Check sheet for the modelled part. Datum: model origin and axes. Units: mm. A direction names the side the tool comes from. Coordinates: 2 decimals unless noted, no trailing zeros. Loops run counter-clockwise (first coordinate to the right, second up) from the corner with the lowest first, then second, coordinate; pieces in that order, holes last. Notation, with made-up numbers: M 44,20 L 56,20 A23 ccw 56,36 Z; hole C 79.5,47 d7. An arc over 180 degrees is marked long. Use CSV: the item, a comma, the result in double quotes. Start each with the question number.
(1) Go/stop test with flat-tipped pins: pin 1 Ø1.6 at (y, z) = (-1, -3.5) entering from +X; pin 2 Ø5 at (x, z) = (12, 5) entering from -Y; pin 3 Ø0.7 at (x, y) = (49, -1) entering from +Z. Record where each tip stops, or that it passes through.
(2) Section check B-B on z = -1. Record the cut outline in (x, y) (3 decimals), and give its area (3 significant figures).
(3) Draft check along Z on faces 4 (the flat face through (62.8, -0.6, -4.3)), 5 (the flat face through (34, -6, -7)), 6 (the cylindrical face through (1.797, -12.913, -6.63)). Enter one of: pulls with the +Z half, pulls with the -Z half, needs draft (parallel to the pull), parting line crosses it, or undercut.
(4) Scan lines: line 1 (Z direction, x = 55.5, y = -2.5); line 2 (Y direction, x = 30, z = 3). Record each from-to range of solid material in increasing order.
(5) Section check C-C on x = 3.95. Give the number of separate pieces and of enclosed holes in the cut face, and give its area (3 significant figures).
(6) Section check A-A on y = -4.3. Record the cut outline in (x, z), and give its area (3 significant figures).
(7) Set-up check for faces 1 (the flat face through (18.986, -11.146, 6.63)), 2 (the flat face through (53, -1, 2.5)), 3 (the flat face through (51.823, -10.222, -6.62)): record each of +Z, -Z, +X, -X, +Y, -Y from which the full face is reachable in a straight line by a thin tool's end or side.
from build123d import *

# Parameters (mm, degrees)
BOSS_EXTRUDE1_DEPTH = 7
FILLET1_R           = 2
FILLET2_R           = 4
SHELL1_T            = -0.75
SKETCH4_R           = 1.5
CUT_EXTRUDE1_DEPTH  = 71.716642035
CUT_EXTRUDE2_DEPTH  = 14
CUT_EXTRUDE3_DEPTH  = 71.716642035


with BuildPart() as part:
    # Sketch3 → Boss-Extrude1 (new, symmetric)
    with BuildSketch(Plane.XY):
        with BuildLine():
            Line((67, 0), (68.2, -9))
            Line((68.2, -9), (1.2, -14))
            Line((1.2, -14), (0, 0))
            ThreePointArc((0, 0), (33.5, -1), (67, 0))
        make_face()
        with BuildLine():
            ThreePointArc((1.2, -14), (-0.147259987, -7.064050856), (0, 0))
            Line((0, 0), (1.2, -14))
        make_face()
    extrude(amount=BOSS_EXTRUDE1_DEPTH, both=True)

    # Fillet1
    fillet1_edges = [part.edges().sort_by_distance(p)[0] for p in [
        (33.5, -1, 7),
        (33.5, -1, -7),
        (68.2, -9, 0),
    ]]
    fillet(fillet1_edges, radius=FILLET1_R)

    # Fillet2
    fillet2_edges = [part.edges().sort_by_distance(p)[0] for p in [
        (1.2, -14, 0),
    ]]
    fillet(fillet2_edges, radius=FILLET2_R)

    # Shell1
    shell1_openings = [part.faces().sort_by_distance(p)[0] for p in [
        (67.467137389, -3.503530417, 0),
        (67.490186671, -8.423793277, 0),
        (1.829469038, -12.937587905, 0),
        (35.321845663, -11.453593607, 0),
        (-0.252281581, -5.271781297, 0),
    ]]
    offset(amount=SHELL1_T, openings=shell1_openings)

    # Sketch4 → Cut-Extrude1 (cut, through all)
    with BuildSketch(Plane.XY.offset(7)):
        with Locations((3.95, -7.3)):
            Circle(SKETCH4_R)
        with Locations((63.05, -4.3)):
            Circle(SKETCH4_R)
    extrude(amount=-CUT_EXTRUDE1_DEPTH, mode=Mode.SUBTRACT)

    # Sketch5 → Cut-Extrude2 (cut)
    with BuildSketch(Plane(origin=(0, 0, 0), x_dir=(1, 0, 0), z_dir=(0, 1, 0))):
        Polygon((17.8, -2), (17.8, 2), (42.8, 2.5), (62.8, 2.5), (62.8, 6.25), (67.8, 6.25), (67.8, -6.25), (62.8, -6.25), (62.8, -2.5), (42.8, -2.5), align=None)
    extrude(amount=-CUT_EXTRUDE2_DEPTH, mode=Mode.SUBTRACT)

    # Sketch6 → Cut-Extrude3 (cut, through all)
    with BuildSketch(Plane.XY.offset(7)):
        with BuildLine():
            Line((18, -12.746268657), (20, -9.5))
            Line((20, -9.5), (30, -9.5))
            ThreePointArc((30, -9.5), (33.691290315, -9.961280118), (37.155551452, -11.316749892))
            Line((37.155551452, -11.316749892), (18, -12.746268657))
        make_face()
    extrude(amount=-CUT_EXTRUDE3_DEPTH, mode=Mode.SUBTRACT)


solid = part.part
Outcome:
1,pin 1,"stops at x = 62.8"
1,pin 2,"stops at y = -13.36"
1,pin 3,"stops at z = 6.39"
2,outline,"M -0.087,-0.746 A562.375 ccw 17.8,-1.531 L 17.8,-0.781 A561.625 cw 0,0 A33.282 ccw Z"
2,area,"13.4 mm²"
3,face 4,"undercut"
3,face 5,"pulls with the -Z half"
3,face 6,"needs draft"
4,line 1,"z = -7 to -6.25, 6.25 to 7"
4,line 2,"y = -1.74 to -0.99"
5,separate pieces,"3"
5,enclosed holes,"0"
5,area,"24.1 mm²"
6,outline,"M -0.27,-7 L 61.55,-7 L 61.55,-6.25 L -0.27,-6.25 Z; M -0.27,6.25 L 61.55,6.25 L 61.55,7 L -0.27,7 Z; M 64.55,-7 L 67.57,-7 L 67.57,-6.25 L 64.55,-6.25 Z; M 64.55,6.25 L 67.57,6.25 L 67.57,7 L 64.55,7 Z"
6,area,"97.3 mm²"
7,face 1,"+Z, -Z, -Y"
7,face 2,"+X, +Y, -Y"
7,face 3,"+Z, -Z, +X, -Y"
